Can you work these out from the model? Positions are in its coordinate system, mm. Face numbers are marked on the shaded views. A direction names the side the tool comes from. Round coordinates to 2 decimals unless told otherwise and drop trailing zeros. Loops run counter-clockwise (first coordinate to the right, second up) from the corner with the lowest first, then second, coordinate; pieces in that order, holes last. Notation, with made-up numbers: (88.5, -4.5) -> (123.5, -4.5) arc R14 cw to (123.5, 1.5) -> close; hole circle Ø8 at (-33, -33). An arc over 180 degrees is marked (long way). Answer as a JSON object with one key per item and string values.
```python
from build123d import *

# Parameters (mm, degrees)
P_IDAT_VYSUNUT_M1_DEPTH  = 30
ODEBRAT_VYSUNUT_M1_REACH = 117.758
SKICA2_W                 = 10
SKICA2_H                 = 10


with BuildPart() as part:
    # Skica1 → Přidat vysunutím1 (new body)
    with BuildSketch(Plane(origin=(0, 0, 0), x_dir=(1, 0, 0), z_dir=(0, 1, 0))):
        Polygon((100, 25), (100, 0), (0, 0), (0, 50), (25, 50), (25, 25), align=None)
    extrude(amount=P_IDAT_VYSUNUT_M1_DEPTH)

    # Skica2 → Odebrat vysunutím1 (cut, up to next)
    with BuildSketch(Plane.XY, mode=Mode.PRIVATE) as odebrat_vysunut_m1_sk1:
        with Locations((95, 25)):
            Rectangle(SKICA2_W, SKICA2_H)
    odebrat_vysunut_m1_tool1 = extrude(odebrat_vysunut_m1_sk1.sketch, amount=-ODEBRAT_VYSUNUT_M1_REACH, mode=Mode.PRIVATE) & part.part
    add(odebrat_vysunut_m1_tool1.solids().sort_by_distance((95, 25, 0))[0], mode=Mode.SUBTRACT)


solid = part.part
```
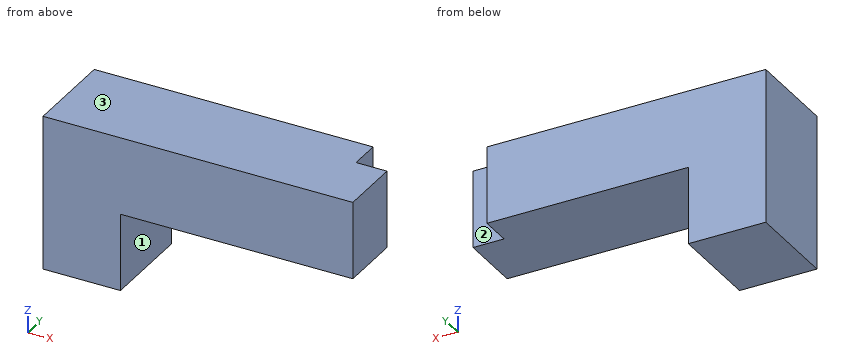
Q1. I'm going to push flat-ended pins straight in: pin 1 (3 mm diameter, centred on y = 25.5, z = -36.5, fed in from +X); pin 2 (4 mm diameter, centred on x = 27.5, y = 8, fed in from -Z); pin 3 (8 mm diameter, centred on x = 95.5, z = -18, fed in from +Y). Where does each tip first touch, or does it pass through?
Determined:
{"pin 1": "x = 25", "pin 2": "z = -25", "pin 3": "y = 20"}
Q2. I want a section at A-A, the plane z = -19. Write out the boundary of the cut face in (x, y).
Determined:
{"outline": "(0, 0) -> (100, 0) -> (100, 20) -> (90, 20) -> (90, 30) -> (0, 30) -> close"}
Q3. If I drill on L1, parallel to X at y = 27.25, z = -4.5; L2, parallel to Z at x = 61.5, y = 5.25; L3, parallel to X at y = 20, z = -35, over which ranges is the centre line in solid material (lowest first)? Write a range as [from, to].
Determined:
{"L1": "[0, 90]", "L2": "[-25, 0]", "L3": "[0, 25]"}
Q4. I want a section at C-C, the plane x = 52. Write out the boundary of the cut face in (y, z).
Determined:
{"outline": "(0, -25) -> (30, -25) -> (30, 0) -> (0, 0) -> close"}
Q5. I want a section at D-D, the plane x = 93. Write out the boundary of the cut face in (y, z).
Determined:
{"outline": "(0, -25) -> (20, -25) -> (20, 0) -> (0, 0) -> close"}
Q6. On a 3-axis mill with a long thin cutter (end or side, diameter ignored), from which of +Z, -Z, +X, -X, +Y, -Y can I reach the whole of each face in a straight line? I mean the marked faces 1, 2 and 3. Say none if no direction works.
Determined:
{"face 1": "-Z, +X, +Y, -Y", "face 2": "+Z, -Z, +X, +Y", "face 3": "+Z, +X, -X, +Y, -Y"}
Q7. I want a section at B-B, the plane y = 28.25. Write out the boundary of the cut face in (x, z).
Determined:
{"outline": "(0, -50) -> (25, -50) -> (25, -25) -> (90, -25) -> (90, 0) -> (0, 0) -> close"}
